Here's how the part is built. I have some questions about the finished solid (model axes, mm). Face numbers are marked on the shaded views. A direction names the side the tool comes from. Coordinates: 2 decimals unless noted, no trailing zeros. Write each loop counter-clockwise with the first axis right and the second up, starting at its lowest first coordinate (ties: lowest second). Pieces come first, ordered by that corner, then holes. Notation, with made-up numbers: (-9, 42) - (12, 42) arc R26 cw to (12, 74) - close; hole circle Ø4 at (35, -3.5). An arc over 180 degrees is marked (long way). Answer in a Markdown table with one row per item. Add a question column.
Item 1: If I drill on probe 1 along Z at (x, y) = (-7.2, 0); probe 2 along Z at (x, y) = (-2.25, -15), over which ranges is the centre line in solid material (lowest first)? Write a range as from..to.
Item 2: Which directions (+Z, -Z, +X, -X, +Y, -Y) give clear straight access to the entire face, cutting with the end or side of a thin tool? Please do the marked faces 1 and 2.
Item 3: We'd pull the mould along Y, two halves only. Please class the marked faces 3, 4 and 5: +Y half, -Y half, draft (parallel to the pull), parting line (faces both ways), or undercut.
Item 4: Imagine slicing it at C-C (y = 15). State how many separate pieces and enclosed holes the cut face has, plus the area to 3 significant figures.
Item 5: Imagine slicing it at B-B (x = -18). Please give me the cut outline in (y, z), plus the area to 3 significant figures.
Item 6: I'm going to push flat-ended pins straight in: pin 1 (1.5 mm diameter, centred on y = 25, z = -3, fed in from -X); pin 2 (8.5 mm diameter, centred on y = 15, z = -25.98, fed in from -X); pin 3 (18.5 mm diameter, centred on y = 6, z = 5.5, fed in from -X); pin 4 (7.5 mm diameter, centred on y = -30, z = 0, fed in from +X). Where does each tip first touch, or does it pass through?
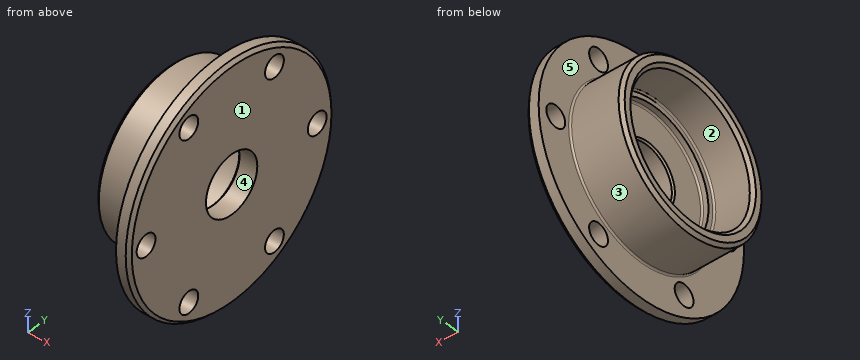
from build123d import *

# Parameters (mm, degrees)
SKETCH_2_W               = 20
SKETCH_2_H               = 9
CHAMFER_1_SIZE           = 1
FILLET_1_R               = 0.5
CHAMFER_2_SIZE           = 0.5
CHAMFER_3_SIZE           = 1
PATTERN_CIRCULAR_1_COUNT = 6


with BuildPart() as part:
    # Эскиз1 → Повернуть1 (revolve)
    with BuildSketch(Plane.XY):
        Polygon((0, 36), (0, 0), (-6, 0), (-6, 19), (-8, 19), (-8, 21), (-20, 21), (-20, 25), (-4, 25), (-4, 36), align=None)
    revolve(axis=Axis((0, 0, 0), (-1, 0, 0)))

    # Эскиз2 → Вырез-Повернуть1 (revolve, cut)
    with BuildSketch(Plane.XY):
        with Locations((-10, 4.5)):
            Rectangle(SKETCH_2_W, SKETCH_2_H)
    revolve(axis=Axis((0, 0, 0), (1, 0, 0)), mode=Mode.SUBTRACT)

    # Фаска1
    chamfer_1_edges = [part.edges().sort_by_distance(p)[0] for p in [
        (-20, -25, 0),
        (-20, -21, 0),
    ]]
    chamfer(chamfer_1_edges, length=CHAMFER_1_SIZE)

    # Скругление1
    fillet_1_edges = [part.edges().sort_by_distance(p)[0] for p in [
        (-6, -19, 0),
        (-4, -25, 0),
        (-8, -21, 0),
    ]]
    fillet(fillet_1_edges, radius=FILLET_1_R)

    # Фаска2
    chamfer_2_edges = [part.edges().sort_by_distance(p)[0] for p in [
        (-6, -9, 0),
    ]]
    chamfer(chamfer_2_edges, length=CHAMFER_2_SIZE)

    # Фаска3
    chamfer_3_edges = [part.edges().sort_by_distance(p)[0] for p in [
        (0, -36, 0),
    ]]
    chamfer(chamfer_3_edges, length=CHAMFER_3_SIZE)

    # Эскиз3 → Отверстие с зазором M61 (revolve, cut)
    with BuildSketch(Plane(origin=(0, -30, 0), x_dir=(0, 0, -1), z_dir=(0, 1, 0))):
        Polygon((0, 0), (0, 17.982840043), (3.3, 16), (3.3, 0), align=None)
    hole_wizard_m61 = revolve(axis=Axis((6.35, -30, 0), (-1, 0, 0)), mode=Mode.SUBTRACT)

    # Круговой массив1: Отверстие с зазором M61 ×6 about axis
    pattern_circular_1_axis = Axis((0, 0, 0), (1, 0, 0))
    for i in range(1, PATTERN_CIRCULAR_1_COUNT):
        add(hole_wizard_m61.rotate(pattern_circular_1_axis, i * 360 / PATTERN_CIRCULAR_1_COUNT), mode=Mode.SUBTRACT)


solid = part.part
Here are the results:
| question | item | result |
|---|---|---|
| 1 | probe 1 | z = -25..-19, 19..25 |
| 1 | probe 2 | z = -32.73..-29.28, -22.68..22.68, 29.28..32.73 |
| 2 | face 1 | +Z, -Z, +X, +Y, -Y |
| 2 | face 2 | -X |
| 3 | face 3 | parting line |
| 3 | face 4 | undercut |
| 3 | face 5 | draft |
| 4 | separate pieces | 3 |
| 4 | enclosed holes | 0 |
| 4 | area | 446 mm2 |
| 5 | outline | circle Ø50 at (0, 0); hole circle Ø42 at (0, 0) |
| 5 | area | 578 mm2 |
| 6 | pin 1 | stops at x = -19.57 |
| 6 | pin 2 | stops at x = -4 |
| 6 | pin 3 | stops at x = -6 |
| 6 | pin 4 | stops at x = 0 |
